Autodesk Inventor part; units mm, degrees
ref_plane "YZ Plane" through (0, 0, 0) normal (1, 0, 0) x (0, 1, 0)
ref_plane "XZ Plane" through (0, 0, 0) normal (0, 1, 0) x (-1, 0, 0)
ref_plane "XY Plane" through (0, 0, 0) normal (0, 0, 1) x (1, 0, 0)
sketch "Sketch2" plane through (0, 0, 0) normal (0, 1, 0) x (-1, 0, 0)
  arc A0 (762, -479.9355) -> (-762, -479.9355) centre (0, 0) ccw
  line L0 (900.5455, 0) -> (762, 0)
  line L1 (762, -479.9355) -> (-762, -479.9355)
  dimension "d8" = 1524
extrude "Extrusion1" add sketch "Sketch2" along normal blind 63.5
sketch "Sketch9" plane through (0, 63.5, 0) normal (0, 1, 0) x (1, 0, 0)
  arc A0 (-762, 479.9355) -> (762, 479.9355) centre (0, 0) ccw
  line L0 (762, 479.9355) -> (-762, 479.9355)
  line L1 (-762, 479.9355) -> (762, 479.9355)
extrude "Extrusion10" add sketch "Sketch9" along normal blind 254
sketch "Sketch10" plane through (0, 317.5, 0) normal (0, 1, 0) x (1, 0, 0)
  arc A0 (-762, 479.9355) -> (762, 479.9355) centre (0, 0) ccw
  line L0 (762, 479.9355) -> (-762, 479.9355)
  line L1 (-762, 479.9355) -> (762, 479.9355)
  arc A1 (-733.4235, 429.1355) -> (733.4235, 429.1355) centre (0, 0) ccw
  line L2 (-733.4235, 429.1355) -> (733.4235, 429.1355)
  line L3 (-733.4235, 429.1355) -> (-791.7227, 429.1355)
  arc A2 (-762, 479.9355) -> (762, 479.9355) centre (0, 0) ccw
  line L4 (733.4235, 429.1355) -> (791.7227, 429.1355)
  line L5 (-794.2175, 302.1355) -> (-848.3491, 302.1355)
  line L6 (-848.381, 48.1355) -> (-899.0048, 48.1355)
  line L7 (-846.0779, -78.8645) -> (-891.7459, -78.8645)
  line L8 (-891.7459, -78.8645) -> (-897.0856, -78.8645)
  line L9 (-899.0048, 48.1355) -> (-899.2581, 48.1355)
  arc A3 (-762, 479.9355) -> (762, 479.9355) centre (0, 0) ccw
  line L10 (-784.9709, -325.4044) -> (-834.8069, -337.7567)
  line L11 (-784.9709, -325.4044) -> (-727.706, -438.7611)
  line L12 (-727.706, -438.7611) -> (-773.1686, -461.7276)
  line L13 (-565.5178, -634.2373) -> (-605.0317, -667.0223)
  line L14 (-565.5178, -634.2373) -> (-464.6758, -711.4378)
  line L15 (-464.6758, -711.4378) -> (-495.6377, -751.8812)
  line L16 (-233.6472, -816.9923) -> (-254.9841, -863.6928)
  line L17 (-109.2742, -842.69) -> (-119.5805, -892.5708)
  line L18 (144.6694, -837.3399) -> (145.7509, -888.6725)
  line L19 (267.8496, -806.4266) -> (280.2477, -855.8291)
  line L20 (494.2276, -691.2354) -> (517.5126, -736.9958)
  line L21 (591.7285, -609.8563) -> (625.6901, -650.5458)
  line L22 (745.5399, -407.7225) -> (786.3996, -438.8142)
  line L23 (797.9796, -292.0545) -> (844.3692, -313.0859)
  line L24 (848.6487, -43.1597) -> (899.5106, -43.1597)
  line L25 (845.6029, 83.8038) -> (896.5226, 85.0253)
  line L26 (783.0573, 329.9827) -> (832.8203, 342.6258)
  point P0 (624.3663, -648.9598)
  dimension "d44" = 50.8
extrude "Extrusion13" cut sketch "Sketch10" against normal blind 254 contours L5 A1 L6 L9 A0 | A0 L25 A1 L26 | L8 L7 A1 L10 A0 | A0 L23 A1 L24 | L12 A1 L13 A0 | A0 L21 A1 L22 | L15 A1 L16 A0 | A0 L19 A1 L20 | L17 A1 L18 A0
sketch "Sketch12" plane through (0, 317.5, 0) normal (0, 1, 0) x (1, 0, 0)
  arc A0 (899.5106, -43.1597) -> (896.5226, 85.0253) centre (0, 0) ccw
  arc A1 (-762, 479.9355) -> (762, 479.9355) centre (0, 0) ccw
  line L0 (762, 479.9355) -> (-762, 479.9355)
  line L1 (-762, 479.9355) -> (762, 479.9355)
  arc A2 (-733.4235, 429.1355) -> (733.4235, 429.1355) centre (0, 0) ccw
  line L2 (-733.4235, 429.1355) -> (733.4235, 429.1355)
  dimension "d73" = 50.8
extrude "Extrusion14" cut sketch "Sketch12" against normal blind 254 contours L2 A2
properties part number "Nest-ver3-1111-2021"
The model under review builds one solid part; all positions refer to its coordinate system, in mm. A direction names the side the tool comes from. Coordinates: 2 decimals unless noted, no trailing zeros. Write each loop counter-clockwise with the first axis right and the second up, starting at its lowest first coordinate (ties: lowest second). Pieces come first, ordered by that corner, then holes. Notation, with made-up numbers: (20.5, -21) -> (59.5, -21) arc R11 cw to (59.5, -7) -> close; hole circle Ø8 at (-34.75, 22). An arc over 180 degrees is marked (long way). One line per item, written item: value. Start each with the question number.
Q1. Add section D-D, the plane y = 32. Give the boundary of the cut face in (x, z), then the cut area to 3 significant figures.
Q2. The part is to be moulded in two halves that separate along Z. For faces 4 (the face through (-517.25, 192.28, 674.18)), 5 (the face through (13, 0, 220)), 6 (the face through (-479.94, 192.278, 731.376)), 7 (the face through (-10, 192, -429.136)), say which applies: +Z half, -Z half, draft (parallel to the pull), parting line (faces both ways), or undercut.
Q3. Add section B-B, the plane x = 0. Give the boundary of the cut face in (y, z).
Q4. To check wall thickness, follow probe 1 along Y at (x, z) = (98.5, 539); probe 2 along Z at (x, y) = (-61, 151); probe 3 along Z at (x, y) = (-546.5, 208.5). State the ranges of each line that lie inside material, in increasing order.
Q5. Add section C-C, the plane y = 291.5. Count the separate pieces of the cut face and the enclosed holes in it, then the cut area to 3 significant figures.
Q6. Clearance check with flat-ended pins moving along their axes: P1, Ø1.5, axis at y = 161, z = 350, coming from the +X side; P2, Ø1.5, axis at x = -331.5, y = 159, coming from the +Z side; P3, Ø15.5, axis at x = 863.5, y = 187.5, coming from the +Z side. State where each tip first meets the part, or that it passes through.
Q7. Add section A-A, the plane z = 0. Give the boundary of the cut face in (x, y).
Q8. For faces 1 (the face through (-821, 192, -302.136)), 2 (the face through (-172.81, 192.28, 831.99)), 3 (the face through (607.819, 192.278, 629.134)), list the 3-axis set-ups (+Z, -Z, +X, -X, +Y, -Y) from which the entire face can be reached by the end or side of a thin tool; tool diameter is ignored.
Response:
1. outline: (-762, -479.94) -> (762, -479.94) arc R900.55 ccw (long way) to start
1. area: 2,100,000 mm²
2. face 4: undercut
2. face 5: draft
2. face 6: +Z half
2. face 7: undercut
3. outline: (0, -479.94) -> (317.5, -479.94) -> (317.5, -429.14) -> (63.5, -429.14) -> (63.5, 900.55) -> (0, 900.55) -> close
4. probe 1: 0 to 63.5
4. probe 2: -479.94 to -429.14
4. probe 3: -479.94 to -429.14, 650.7 to 715.77
5. separate pieces: 9
5. enclosed holes: 0
5. area: 145,000 mm²
6. P1: x = 830.06
6. P2: z = -429.14
6. P3: z = 43.16
7. outline: (-900.55, 0) -> (900.55, 0) -> (900.55, 317.5) -> (849.75, 317.5) -> (849.75, 63.5) -> (-849.75, 63.5) -> (-849.75, 317.5) -> (-900.55, 317.5) -> close
8. face 1: +X, -X, +Y
8. face 2: +Y
8. face 3: +X, +Y
